```python
from build123d import *

# Parameters (mm, degrees)
SKETCH1_W           = 82.55
SKETCH1_H           = 26.67
BOSS_EXTRUDE1_DEPTH = 1.5875
SKETCH2_R           = 1.651
SKETCH2_R_2         = 1.5875
CUT_EXTRUDE1_DEPTH  = 3.175
SKETCH5_W           = 82.55
SKETCH5_H           = 3.175
BOSS_EXTRUDE3_DEPTH = 27.94
SKETCH6_R           = 1.524
CUT_EXTRUDE3_DEPTH  = 3.175
CUT_EXTRUDE4_DEPTH  = 3.175
BOSS_EXTRUDE4_DEPTH = 82.55
CUT_EXTRUDE5_DEPTH  = 3.175
SKETCH10_W          = 9.525
SKETCH10_H          = 82.55
BOSS_EXTRUDE5_DEPTH = 2.286


with BuildPart() as part:
    # Sketch1 → Boss-Extrude1 (new, symmetric)
    with BuildSketch(Plane(origin=(0, 0, 0), x_dir=(0, 0, -1), z_dir=(1, 0, 0))):
        Rectangle(SKETCH1_W, SKETCH1_H)
    extrude(amount=BOSS_EXTRUDE1_DEPTH, both=True)

    # Sketch2 → Cut-Extrude1 (cut)
    with BuildSketch(Plane.ZY.offset(1.5875)):
        with Locations((33.3375, -5.715)):
            Circle(SKETCH2_R)
        with Locations((-33.3375, -5.715)):
            Circle(SKETCH2_R)
        with Locations((-26.4795, -10.16)):
            Circle(SKETCH2_R_2)
        with Locations((26.4795, -10.16)):
            Circle(SKETCH2_R_2)
    extrude(amount=-CUT_EXTRUDE1_DEPTH, mode=Mode.SUBTRACT)

    # Sketch5 → Boss-Extrude3 (add)
    with BuildSketch(Plane.ZY.offset(1.5875)):
        with Locations((0, 14.9225)):
            Rectangle(SKETCH5_W, SKETCH5_H)
    extrude(amount=-BOSS_EXTRUDE3_DEPTH)

    # Sketch6 → Cut-Extrude3 (cut)
    with BuildSketch(Plane(origin=(0, 16.51, 0), x_dir=(1, 0, 0), z_dir=(0, 1, 0))):
        with Locations(Location((17.4625, 19.05, 0), (0, 0, 270))):
            Circle(SKETCH6_R)
        with Locations(Location((17.4625, -19.05, 0), (0, 0, 270))):
            Circle(SKETCH6_R)
    extrude(amount=-CUT_EXTRUDE3_DEPTH, mode=Mode.SUBTRACT)

    # Sketch7 → Cut-Extrude4 (cut)
    with BuildSketch(Plane.ZY.offset(1.5875)):
        Polygon((-31.75, -13.335), (31.75, -13.335), (27.94, -5.207), (-27.94, -5.207), align=None)
    extrude(amount=-CUT_EXTRUDE4_DEPTH, mode=Mode.SUBTRACT)

    # Sketch8 → Boss-Extrude4 (add)
    with BuildSketch(Plane.XY.offset(41.275)):
        Polygon((1.5875, 13.335), (9.2075, 13.335), (1.5875, 5.715), align=None)
    extrude(amount=-BOSS_EXTRUDE4_DEPTH)

    # Sketch9 → Cut-Extrude5 (cut)
    with BuildSketch(Plane.ZY.offset(1.5875)):
        Polygon((-41.275, -13.335), (-41.275, -9.525), (-29.9640625, -9.525), (-31.75, -13.335), align=None)
        Polygon((41.275, -13.335), (41.275, -9.525), (29.9640625, -9.525), (31.75, -13.335), align=None)
    extrude(amount=-CUT_EXTRUDE5_DEPTH, mode=Mode.SUBTRACT)

    # Sketch10 → Boss-Extrude5 (add)
    with BuildSketch(Plane(origin=(0, 16.51, 0), x_dir=(1, 0, 0), z_dir=(0, 1, 0))):
        with Locations((3.175, 0)):
            Rectangle(SKETCH10_W, SKETCH10_H)
    extrude(amount=BOSS_EXTRUDE5_DEPTH)


solid = part.part
```
Source: CAD feature listing. Evaluate the final solid. Frame: model axes, mm. A direction names the side the tool comes from. Give positions to 0.01 mm unless a question says otherwise; leave off trailing zeros. Write each loop counter-clockwise with the first axis right and the second up, starting at its lowest first coordinate (ties: lowest second). Pieces come first, ordered by that corner, then holes.
1. Section query A-A (z = -7.5). Return the cut outline in (x, y) (1 decimal), then the cut area to 3 significant figures.
2. Section query C-C (y = 2.25). Return the cut outline in (x, z) (1 decimal), then the cut area to 3 significant figures.
3. Section query D-D (x = 4.75). Return the cut outline in (y, z) (1 decimal).
4. Section query B-B (z = 19.05). Return the cut outline in (x, y) (1 decimal).
5. Access query for faces 1 (the face through (-0.02, -7.34, -28.94)), 2 (the face through (0, -9.525, 36)), 3 (the face through (-0.022, -5.219, 34.912)), 4 (the face through (1.588, 0, 1)), 5 (the face through (7.938, 18, 1)). Directions: +Z, -Z, +X, -X, +Y, -Y. A direction counts if a zero-diameter tool reaches every point of the face in a straight line with its end or side. Return the directions, or none.
6. Material intervals for line 1 along X through (y, z) = (15.4, -19.05); line 2 along Y through (x, z) = (17.5, -7.5) (3 decimals); line 3 along X through (y, z) = (-3.5, 25), sorted ascending.
7. First-contact query: pin 1 (1 mm diameter, centred on y = 9.5, z = -32.5, fed in from +X); pin 2 (8 mm diameter, centred on x = 13.5, z = -9.5, fed in from -Y) (3 decimals); pin 3 (7.5 mm diameter, centred on y = -3.5, z = 3, fed in from +X). Flat tips, straight axial feed; report the tip coordinate or a pass-through.
8. Pull-direction query (Y, two-part tool) for faces 6 (the face through (-0.022, -5.219, -31.763)), 7 (the face through (18, 13.335, -1)), 8 (the face through (26.353, 15, -1)); classes: +Y half, -Y half, draft (parallel to the pull), parting line (faces both ways), or undercut.
Output values:
1. outline: (-1.6, -5.2) - (1.6, -5.2) - (1.6, 5.7) - (9.2, 13.3) - (26.4, 13.3) - (26.4, 16.5) - (7.9, 16.5) - (7.9, 18.8) - (-1.6, 18.8) - close
1. area: 198 mm2
2. outline: (-1.6, -41.3) - (1.6, -41.3) - (1.6, 41.3) - (-1.6, 41.3) - close
2. area: 262 mm2
3. outline: (8.9, -41.3) - (18.8, -41.3) - (18.8, 41.3) - (8.9, 41.3) - close
4. outline: (-1.6, -5.2) - (1.6, -5.2) - (1.6, 5.7) - (9.2, 13.3) - (15.9, 13.3) - (15.9, 16.5) - (7.9, 16.5) - (7.9, 18.8) - (-1.6, 18.8) - close; (19, 13.3) - (26.4, 13.3) - (26.4, 16.5) - (19, 16.5) - close
5. face 1: +X, -X, -Y
5. face 2: +Z, -Z, +X, -X, -Y
5. face 3: +X, -X
5. face 4: +Z, -Z, +X, -Y
5. face 5: +Z, -Z, +X, +Y
6. line 1: x = -1.59 to 15.94, 18.99 to 26.35
6. line 2: y = 13.335 to 16.51
6. line 3: x = -1.59 to 1.59
7. pin 1: stops at x = 5.87
7. pin 2: stops at y = 13.335
7. pin 3: stops at x = 1.59
8. face 6: undercut
8. face 7: -Y half
8. face 8: draft
